Can you work these out from the model? Positions are in its coordinate system, mm. Face numbers are marked on the shaded views. A direction names the side the tool comes from. Round coordinates to 2 decimals unless told otherwise and drop trailing zeros. Loops run counter-clockwise (first coordinate to the right, second up) from the corner with the lowest first, then second, coordinate; pieces in that order, holes last.
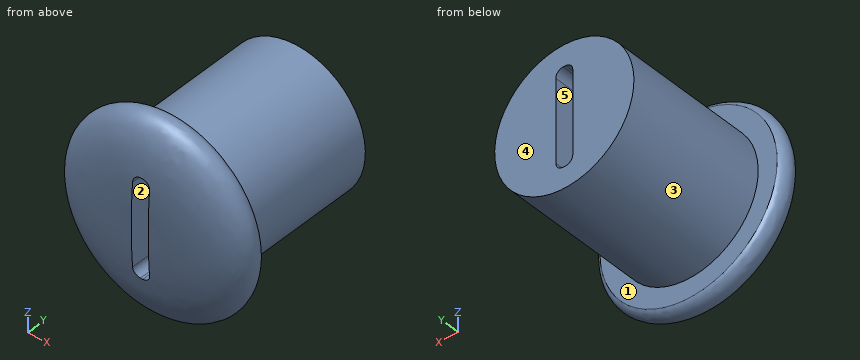
```python
from build123d import *

# Parameters (mm, degrees)
F3_DEPTH = 25.0491994545


with BuildPart() as f1:
    # F0 (on Right) → F1 (revolve)
    with BuildSketch(Plane.YZ):
        with BuildLine():
            Line((-25, 0), (0, 0))
            Line((0, 0), (0, 9.5))
            Line((0, 9.5), (-20, 9.5))
            Line((-20, 9.5), (-20, 12.0843162353))
            add(Edge.make_bspline(
                [(-25, 0), (-25.0620774302, 2.5433010343), (-25.0716983516, 3.4419194063), (-24.5929996185, 10.3825960783), (-21.9290160892, 13.4230087933), (-20.1981659595, 12.6572140375), (-20, 12.0843162353)],
                knots=[0, 0, 0, 0, 0.2637629191, 0.5846935152, 0.8278932887, 1, 1, 1, 1], degree=3))
        make_face()
    revolve(axis=Axis((0, -12.5, 0), (0, -1, 0)))

    # F2 (on face) → F3 (cut, through all)
    with BuildSketch(Plane(origin=(0, 0, 0), x_dir=(-1, 0, 0), z_dir=(0, 1, 0))):
        with BuildLine():
            ThreePointArc((1.1575235985, 5.6240597516), (0.8646303797, 6.3311665328), (0.1575235985, 6.6240597516))
            Line((0.1575235985, 6.6240597516), (-0.1575235985, 6.6240597516))
            ThreePointArc((-0.1575235985, 6.6240597516), (-0.8646303797, 6.3311665328), (-1.1575235985, 5.6240597516))
            Line((-1.1575235985, 5.6240597516), (-1.1575235985, -5.6240597516))
            ThreePointArc((-1.1575235985, -5.6240597516), (-0.8646303797, -6.3311665328), (-0.1575235985, -6.6240597516))
            Line((-0.1575235985, -6.6240597516), (0.1575235985, -6.6240597516))
            ThreePointArc((0.1575235985, -6.6240597516), (0.8646303797, -6.3311665328), (1.1575235985, -5.6240597516))
            Line((1.1575235985, -5.6240597516), (1.1575235985, 5.6240597516))
        make_face()
    extrude(amount=-F3_DEPTH, mode=Mode.SUBTRACT)


solid = f1.part
```
(1) Suppose I cut it at A-A (y = -10). Write out the boundary of the cut face in (x, z), then the cut area to 3 significant figures.
(2) We'd pull the mould along Z, two halves only. Please class the marked faces 3, 4 and 5: released by +Z, released by -Z, zero draft, split by the parting line, or undercut.
(3) If I drill on line 1 (Z direction, x = 0.25, y = -5.25); line 2 (X direction, y = -23.25, z = -3.25); line 3 (Z direction, x = 1, y = -4), over which ranges is the centre line in solid material (lowest first)?
(4) For pin 1 (1 mm diameter, centred on x = -3.5, y = -10, fed in from -Z); pin 2 (6 mm diameter, centred on x = 7, z = -9.5, fed in from -Y); pin 3 (1 mm diameter, centred on x = -7.5, y = -18.5, fed in from -Z), each with a flat end and sliding along its axis, tell me the tip position at first contact or that it passes through.
(5) Which directions (+Z, -Z, +X, -X, +Y, -Y) give clear straight access to the entire face, cutting with the end or side of a thin tool? Please do the marked faces 1 and 2.
Check result:
1. outline: circle Ø19 at (0, 0); hole (-1.16, -5.62) arc R1 ccw to (-0.16, -6.62) - (0.16, -6.62) arc R1 ccw to (1.16, -5.62) - (1.16, 5.62) arc R1 ccw to (0.16, 6.62) - (-0.16, 6.62) arc R1 ccw to (-1.16, 5.62) - close
1. area: 254 mm2
2. face 3: split by the parting line
2. face 4: zero draft
2. face 5: undercut
3. line 1: z = -9.5 to -6.62, 6.62 to 9.5
3. line 2: x = -11.2 to -1.16, 1.16 to 11.2
3. line 3: z = -9.45 to -6.16, 6.16 to 9.45
4. pin 1: stops at z = -9.01
4. pin 2: stops at y = -24.43
4. pin 3: stops at z = -6.42
5. face 1: +Y
5. face 2: +Y, -Y
